Geometry: final body of the model. Coordinates: model frame, mm. Coordinates: 2 decimals unless noted, no trailing zeros. Write each loop counter-clockwise with the first axis right and the second up, starting at its lowest first coordinate (ties: lowest second). Pieces come first, ordered by that corner, then holes. Notation, with made-up numbers: (-33, 0) - (19, 0) arc R11 ccw to (19, 12) - close; hole circle Ø10 at (89, 29). An arc over 180 degrees is marked (long way). Put each result on its own line as item: value.
```python
from build123d import *

# Parameters (mm, degrees)
STOCK_GEARBOX_START                           = 12.7
STOCK_GEARBOX_WHEEL_PROTOTYPE_STRUCT_2_W      = 76.2
STOCK_GEARBOX_WHEEL_PROTOTYPE_STRUCT_2_H      = 101.6
STOCK_GEARBOX_WHEEL_PROTOTYPE_STRUCT_2_R      = 2.5527
STOCK_GEARBOX_WHEEL_PROTOTYPE_STRUCT_2_R_2    = 2.0193
STOCK_GEARBOX_WHEEL_PROTOTYPE_STRUCT_2_R_3    = 32.5
STOCK_GEARBOX_WHEEL_PROTOTYPE_STRUCTURE_DEPTH = 6.35
SKETCH1_R                                     = 32.754
CUT_EXTRUDE1_DEPTH                            = 64.816710194


# Read off the part's stored shape, not the designer's step: Stock-Gearbox Wheel Prototype Structure-1
with BuildPart() as part:
    # Stock-Gearbox Wheel Prototype Struct 2 → Stock-Gearbox Wheel Prototype Structure-1 (new body)
    with BuildSketch(Plane(origin=(0, 0, 0), x_dir=(1, 0, 0), z_dir=(0, 1, 0)).offset(STOCK_GEARBOX_START)):
        Rectangle(STOCK_GEARBOX_WHEEL_PROTOTYPE_STRUCT_2_W, STOCK_GEARBOX_WHEEL_PROTOTYPE_STRUCT_2_H)
        with Locations((-31.75, -44.45)):
            Circle(STOCK_GEARBOX_WHEEL_PROTOTYPE_STRUCT_2_R, mode=Mode.SUBTRACT)
        with Locations((-25.226034419, -25.226034419)):
            Circle(STOCK_GEARBOX_WHEEL_PROTOTYPE_STRUCT_2_R_2, mode=Mode.SUBTRACT)
        with Locations((31.75, -44.45)):
            Circle(STOCK_GEARBOX_WHEEL_PROTOTYPE_STRUCT_2_R, mode=Mode.SUBTRACT)
        Circle(STOCK_GEARBOX_WHEEL_PROTOTYPE_STRUCT_2_R_3, mode=Mode.SUBTRACT)
        with Locations((25.226034419, -25.226034419)):
            Circle(STOCK_GEARBOX_WHEEL_PROTOTYPE_STRUCT_2_R_2, mode=Mode.SUBTRACT)
        with Locations((-25.226034419, 25.226034419)):
            Circle(STOCK_GEARBOX_WHEEL_PROTOTYPE_STRUCT_2_R_2, mode=Mode.SUBTRACT)
        with Locations((-31.75, 44.45)):
            Circle(STOCK_GEARBOX_WHEEL_PROTOTYPE_STRUCT_2_R, mode=Mode.SUBTRACT)
        with Locations((25.226034419, 25.226034419)):
            Circle(STOCK_GEARBOX_WHEEL_PROTOTYPE_STRUCT_2_R_2, mode=Mode.SUBTRACT)
        with Locations((31.75, 44.45)):
            Circle(STOCK_GEARBOX_WHEEL_PROTOTYPE_STRUCT_2_R, mode=Mode.SUBTRACT)
    extrude(amount=STOCK_GEARBOX_WHEEL_PROTOTYPE_STRUCTURE_DEPTH)

    # Sketch1 → Cut-Extrude1 (cut, through all)
    with BuildSketch(Plane(origin=(0, 19.05, 0), x_dir=(1, 0, 0), z_dir=(0, 1, 0))):
        with Locations(Location((0, 0, 0), (0, 0, 270))):
            Circle(SKETCH1_R)
    extrude(amount=-CUT_EXTRUDE1_DEPTH, mode=Mode.SUBTRACT)


solid = part.part
```
1. Section query B-B (z = 0). Return loops of the section in (x, y), then the cut area to 3 significant figures.
Answer below:
outline: (-38.1, 12.7) - (-32.75, 12.7) - (-32.75, 19.05) - (-38.1, 19.05) - close; (32.75, 12.7) - (38.1, 12.7) - (38.1, 19.05) - (32.75, 19.05) - close
area: 67.9 mm²
2. Section query A-A (z = -44.45). Return loops of the section in (x, y).
Answer below:
outline: (-38.1, 12.7) - (-34.3, 12.7) - (-34.3, 19.05) - (-38.1, 19.05) - close; (-29.2, 12.7) - (29.2, 12.7) - (29.2, 19.05) - (-29.2, 19.05) - close; (34.3, 12.7) - (38.1, 12.7) - (38.1, 19.05) - (34.3, 19.05) - close
3. Mould query, pull axis Z, two halves, no side actions, for faces 1 (the cylindrical face through (34.185, 15.831, -45.217)), 2 (the flat face through (-1, 16, -50.8)), 3 (the cylindrical face through (23.62, 15.83, -24)), 4 (the flat face through (-34, 19.05, -1)). Classes: +Z half, -Z half, draft (parallel to the pull), parting line (faces both ways), or undercut.
Answer below:
face 1: undercut
face 2: -Z half
face 3: undercut
face 4: draft
4. Section query C-C (x = 0). Return loops of the section in (y, z).
Answer below:
outline: (12.7, -50.8) - (19.05, -50.8) - (19.05, -32.75) - (12.7, -32.75) - close; (12.7, 32.75) - (19.05, 32.75) - (19.05, 50.8) - (12.7, 50.8) - close
5. Section query D-D (y = 18). Count the separate pieces of the cut face and the enclosed holes in it, then the cut area to 3 significant figures.
Answer below:
separate pieces: 1
enclosed holes: 9
area: 4,240 mm²
6. Ray query, probe 1 along X at (y, z) = (16, -44.45); probe 2 along X at (y, z) = (13.5, -0.5); probe 3 along Z at (x, y) = (25.5, 18). Return the intervals inside material, ascending. Write a range as from..to.
Answer below:
probe 1: x = -38.1..-34.3, -29.2..29.2, 34.3..38.1
probe 2: x = -38.1..-32.75, 32.75..38.1
probe 3: z = -50.8..-27.23, -23.23..-20.56, 20.56..23.23, 27.23..50.8
